Geometry: final body of the model. Coordinates: model frame, mm. A direction names the side the tool comes from. Coordinates: 2 decimals unless noted, no trailing zeros. Order: outer loops, then holes, each group sorted by start corner. A loop starts at its lowest first (then second) coordinate and runs counter-clockwise, first axis right, second up. Notation, with made-up numbers: M 32,-11 L 41,-11 A5 ccw 41,-7 Z; hole C -14,13.25 d4. An arc over 180 degrees is marked long. Write item = value, one per line.
from build123d import *

# Parameters (mm, degrees)
F0_W     = 50.8
F0_H     = 50.8
F1_DEPTH = 50.8
F3_DEPTH = 2.54
F5_DEPTH = 2.54
F7_DEPTH = 2.54
F9_DEPTH = 2.54


with BuildPart() as f1:
    # F0 (on Front) → F1 (new body)
    with BuildSketch(Plane.XZ):
        with Locations((-4.556354, -11.571446)):
            Rectangle(F0_W, F0_H)
    extrude(amount=F1_DEPTH)

    # F2 (on face) → F3 (cut)
    with BuildSketch(Plane.XY.offset(13.828554)):
        Polygon((-24.876354, -12.728567), (-29.956354, -12.728567), (-29.956354, -50.8), (20.843646, -50.8), (20.843646, -12.728567), (15.763646, -12.728567), (15.763646, -22.888567), (10.683646, -22.888567), (10.683646, -17.808567), (5.603646, -17.808567), (5.603646, -12.728567), (0.523646, -12.728567), (0.523646, -17.808567), (-4.556354, -17.808567), (-4.556354, -12.728567), (-9.636354, -12.728567), (-14.716354, -12.728567), (-14.716354, -7.648567), (-19.796354, -7.648567), (-19.796354, -17.808567), (-24.876354, -17.808567), align=None)
    extrude(amount=-F3_DEPTH, mode=Mode.SUBTRACT)

    # F4 (on face) → F5 (cut)
    with BuildSketch(Plane.YZ.offset(20.843646)):
        Polygon((-12.728567, 8.748554), (-12.728567, 11.288554), (-50.8, 11.288554), (-50.8, -36.971446), (-12.728567, -36.971446), (-12.728567, -31.891446), (-17.808567, -31.891446), (-17.808567, -26.811446), (-12.728567, -26.811446), (-12.728567, -21.731446), (-7.648567, -21.731446), (-7.648567, -16.651446), (-12.728567, -16.651446), (-17.808567, -16.651446), (-17.808567, -11.571446), (-12.728567, -11.571446), (-12.728567, -6.491446), (-22.888567, -6.491446), (-22.888567, -1.411446), (-17.808567, -1.411446), (-17.808567, 3.668554), (-17.808567, 8.748554), align=None)
    extrude(amount=-F5_DEPTH, mode=Mode.SUBTRACT)

    # F6 (on face) → F7 (cut)
    with BuildSketch(Plane(origin=(0, 0, -36.971446), x_dir=(1, 0, 0), z_dir=(0, 0, -1))):
        Polygon((15.763646, 12.728567), (18.303646, 12.728567), (18.303646, 50.8), (-29.956354, 50.8), (-29.956354, 22.881104), (-24.876354, 22.881104), (-24.876354, 17.801104), (-19.796354, 17.801104), (-19.796354, 7.648567), (-14.716354, 7.648567), (-14.716354, 17.801104), (-9.636354, 17.801104), (-9.636354, 12.728567), (-4.556354, 12.728567), (-4.556354, 17.801104), (0.523646, 17.801104), (0.523646, 12.728567), (5.603646, 12.728567), (5.603646, 7.648567), (10.683646, 7.648567), (10.683646, 12.728567), (10.683646, 17.801104), (15.763646, 17.801104), align=None)
    extrude(amount=-F7_DEPTH, mode=Mode.SUBTRACT)

    # F8 (on face) → F9 (cut)
    with BuildSketch(Plane(origin=(-29.956354, 0, 0), x_dir=(0, -1, 0), z_dir=(-1, 0, 0))):
        Polygon((22.881104, -31.891446), (22.881104, -34.431446), (50.8, -34.431446), (50.8, 11.288554), (12.728567, 11.288554), (12.728567, 13.828554), (12.721104, 3.668554), (17.801104, 3.668554), (17.801104, -1.411446), (22.881104, -1.411446), (22.881104, -6.491446), (17.801104, -6.491446), (17.801104, -11.571446), (17.801104, -16.651446), (12.721104, -16.651446), (12.721104, -26.811446), (17.801104, -26.811446), (17.801104, -31.891446), align=None)
    extrude(amount=-F9_DEPTH, mode=Mode.SUBTRACT)


solid = f1.part
1) Section C-C, the plane y = -31. Return loops of the section in (x, z).
Numbers:
outline = M -27.42,-34.43 L 18.3,-34.43 L 18.3,11.29 L -27.42,11.29 Z
2) Section A-A, the plane x = 9.5. Return loops of the section in (y, z).
Numbers:
outline = M -50.8,-34.43 L -7.65,-34.43 L -7.65,-36.97 L 0,-36.97 L 0,13.83 L -17.81,13.83 L -17.81,11.29 L -50.8,11.29 Z
3) Pin query (flat end, axial travel): pin 1 (0.8 mm diameter, centred on y = -14, z = 13, fed in from +X); pin 2 (0.8 mm diameter, centred on x = 20, z = 3, fed in from -Y); pin 3 (1 mm diameter, centred on x = 8, y = -29.5, fed in from +Z). Return the tip coordinate at first contact, or that it passes through.
Numbers:
pin_1 = 15.76
pin_2 = -17.81
pin_3 = 11.29
4) Line query: L1, parallel to Z at x = -12.5, y = -48; L2, parallel to X at y = -23, z = -12.5; L3, parallel to Z at x = 10, y = -13. Output: solid intervals per line, ascending.
Numbers:
L1 = -34.43 to 11.29
L2 = -27.42 to 18.3
L3 = -34.43 to 13.83
5) Set-up query: faces 4 (the face through (20, -15, -11.571)), 5 (the face through (-24.876, -20, -36)), 6 (the face through (20, -15, 8.749)), 7 (the face through (-2, -17.809, 13)), 8 (the face through (10.684, -13, -36)). Return all of +Z, -Z, +X, -X, +Y, -Y with unobstructed straight access to the full face (end or side cutting, diameter ignored); none if empty.
Numbers:
face_4 = +X, -Y
face_5 = -Z, +X, -Y
face_6 = +Z, +X, -Y
face_7 = +Z, -X, -Y
face_8 = -Z, -Y
6) Mould query, pull axis Z, two halves, no side actions, for faces 1 (the face through (20, -20, -1.411)), 2 (the face through (-10, -12.729, 13)), 3 (the face through (20, -15, -26.811)). Classes: pulls with the +Z half, pulls with the -Z half, needs draft (parallel to the pull), parting line crosses it, or undercut.
Numbers:
face_1 = pulls with the +Z half
face_2 = needs draft
face_3 = undercut
7) Section B-B, the plane z = -20.5. Return loops of the section in (x, y), and give its area (3 significant figures).
Numbers:
outline = M -29.96,-12.72 L -27.42,-12.72 L -27.42,-50.8 L 18.3,-50.8 L 18.3,-7.65 L 20.84,-7.65 L 20.84,0 L -29.96,0 Z
area = 2,370 mm²
